Source: CAD feature listing. Evaluate the final solid. Frame: model axes, mm. A direction names the side the tool comes from. Round coordinates to 2 decimals unless told otherwise and drop trailing zeros. Loops run counter-clockwise (first coordinate to the right, second up) from the corner with the lowest first, then second, coordinate; pieces in that order, holes last. Notation, with made-up numbers: (67.5, -14) -> (90.5, -14) arc R31 cw to (90.5, 25) -> close; hole circle Ø11 at (6, 46). An arc over 180 degrees is marked (long way). Return JSON: item names as keys, results as strings. Group by question number.
```python
from build123d import *

# Parameters (mm, degrees)
SKETCH_W        = 9
SKETCH_H        = 10.5
PAD_DEPTH       = 9
POCKET_DEPTH    = 8
PAD001_DEPTH    = 1
SKETCH004_W     = 2
SKETCH004_H     = 6
POCKET002_DEPTH = 1.5
SKETCH007_R     = 1.8
POCKET011_DEPTH = 10.001
POCKET012_DEPTH = 1
SKETCH033_W     = 2
SKETCH033_H     = 1
POCKET013_DEPTH = 1


with BuildPart() as part:
    # Sketch → Pad (new body)
    with BuildSketch(Plane.XY):
        with Locations((0, 0.75)):
            Rectangle(SKETCH_W, SKETCH_H)
    extrude(amount=PAD_DEPTH)

    # Sketch001 (on Face5 of Pad) → Pocket (cut)
    with BuildSketch(Plane(origin=(0, 0, 0), x_dir=(1, 0, 0), z_dir=(0, 0, -1))):
        Polygon((-3.75, 3.63), (-3.75, 3.13), (-2.75, 3.13), (-2.75, 1.13), (-3.75, 1.13), (-3.75, -3.67), (-2.75, -3.67), (-2.75, -4.67), (-3.75, -4.67), (-3.75, -5.17), (3.75, -5.17), (3.75, -4.67), (2.75, -4.67), (2.75, -3.67), (3.75, -3.67), (3.75, 1.13), (2.75, 1.13), (2.75, 3.13), (3.75, 3.13), (3.75, 3.63), align=None)
    extrude(amount=-POCKET_DEPTH, mode=Mode.SUBTRACT)

    # Sketch002 (on Face5 of Pocket) → Pad001 (join)
    with BuildSketch(Plane.XY.offset(9)):
        with BuildLine():
            Line((-2.25, 3), (2.25, 3))
            ThreePointArc((2.25, -3), (3.75, 0), (2.25, 3))
            Line((2.25, -3), (-2.25, -3))
            ThreePointArc((-2.25, 3), (-3.75, 0), (-2.25, -3))
        make_face()
    extrude(amount=PAD001_DEPTH)

    # Sketch004 → Pocket002 (cut)
    with BuildSketch(Plane(origin=(0, 6, 0), x_dir=(-1, 0, 0), z_dir=(0, 1, 0))):
        with Locations((0, 6)):
            Rectangle(SKETCH004_W, SKETCH004_H)
    extrude(amount=-POCKET002_DEPTH, mode=Mode.SUBTRACT)

    # Sketch007 → Pocket011 (cut, through all)
    with BuildSketch(Plane(origin=(0, 0, 10), x_dir=(1, 0, 0), z_dir=(0, 0, -1))):
        Circle(SKETCH007_R)
    extrude(amount=POCKET011_DEPTH, mode=Mode.SUBTRACT)

    # Sketch032 (on Face9 of Pocket011) → Pocket012 (cut)
    with BuildSketch(Plane.XZ.offset(4.5)):
        Polygon((-3, 9), (-3, 6), (-1, 6), (-1, 3.5), (1, 3.5), (1, 6), (3, 6), (3, 9), align=None)
    extrude(amount=-POCKET012_DEPTH, mode=Mode.SUBTRACT)

    # Sketch033 (on Face31 of Pocket012) → Pocket013 (cut)
    with BuildSketch(Plane.XZ.offset(3.5)):
        with Locations((0, 8.5)):
            Rectangle(SKETCH033_W, SKETCH033_H)
    extrude(amount=-POCKET013_DEPTH, mode=Mode.SUBTRACT)


solid = part.part
```
(1) Cut plane D-D (y = 4). Return loops of the section in (x, z), and give its area (3 significant figures).
(2) Ray query, line 1 (Y direction, x = -3.5, z = 5.25); line 2 (Y direction, x = -0.25, z = 2.5); line 3 (Y direction, x = 0, z = 8.7). Return the intervals inside material, ascending.
(3) Cut plane C-C (z = 9.25). Return loops of the section in (x, y).
(4) Cut plane B-B (y = 0). Return loops of the section in (x, z), and give its area (3 significant figures).
(5) Mould query, pull axis Y, two halves, no side actions, for faces 1 (the face through (-3, -1.13, 4)), 2 (the face through (-3, -2, 0)), 3 (the face through (-2, -3.5, 8.5)). Classes: released by +Y, released by -Y, zero draft, split by the parting line, or undercut.
(6) Cut plane A-A (x = 0). Return loops of the section in (y, z).
(7) Pin query (flat end, axial travel): pin 1 (1.1 mm diameter, centred on x = 0, z = 8.5, fed in from -Y); pin 2 (5 mm diameter, centred on x = 1.5, y = -2.5, fed in from -Z); pin 3 (4 mm diameter, centred on x = -1, y = 0, fed in from -Z); pin 4 (1.1 mm diameter, centred on x = -1.5, z = 8.5, fed in from -Y). Return the tip coordinate at first contact, or that it passes through.
(8) Set-up query: faces 4 (the face through (0, -2.5, 8.5)), 5 (the face through (3.75, 1, 4)), 6 (the face through (2, -3.5, 8.5)), 7 (the face through (1, -4, 5)). Return all of +Z, -Z, +X, -X, +Y, -Y with unobstructed straight access to the full face (end or side cutting, diameter ignored); none if empty.
Answers follow:
{
 "1": {"outline": "(-4.5, 0) -> (-2.75, 0) -> (-2.75, 8) -> (2.75, 8) -> (2.75, 0) -> (4.5, 0) -> (4.5, 9) -> (-4.5, 9) -> close", "area": "37.0 mm^2"},
 "2": {"line 1": "-4.5 to -3.63, -3.13 to -1.13, 3.67 to 4.67, 5.17 to 6", "line 2": "-4.5 to -3.63, 5.17 to 6", "line 3": "-2.5 to -1.8, 1.8 to 4.5"},
 "3": {"outline": "(-2.25, -3) -> (2.25, -3) arc R3.75 ccw to (2.25, 3) -> (-2.25, 3) arc R3.75 ccw to start; hole circle Ø3.6 at (0, 0)"},
 "4": {"outline": "(-4.5, 0) -> (-3.75, 0) -> (-3.75, 8) -> (-1.8, 8) -> (-1.8, 10) -> (-3.75, 10) -> (-3.75, 9) -> (-4.5, 9) -> close; (1.8, 8) -> (3.75, 8) -> (3.75, 0) -> (4.5, 0) -> (4.5, 9) -> (3.75, 9) -> (3.75, 10) -> (1.8, 10) -> close", "area": "21.3 mm^2"},
 "5": {"face 1": "undercut", "face 2": "zero draft", "face 3": "released by -Y"},
 "6": {"outline": "(-4.5, 0) -> (-3.63, 0) -> (-3.63, 3.5) -> (-4.5, 3.5) -> close; (-3, 9) -> (-2.5, 9) -> (-2.5, 8) -> (-1.8, 8) -> (-1.8, 10) -> (-3, 10) -> close; (1.8, 8) -> (4.5, 8) -> (4.5, 9) -> (3, 9) -> (3, 10) -> (1.8, 10) -> close; (5.17, 0) -> (6, 0) -> (6, 3) -> (5.17, 3) -> close"},
 "7": {"pin 1": "y = -3", "pin 2": "z = 0", "pin 3": "z = 8", "pin 4": "y = -3.5"},
 "8": {"face 4": "-Z, -Y", "face 5": "-Z", "face 6": "+Z, -Z, -Y", "face 7": "+Z, +Y, -Y"}
}
